Read the model definition and answer for the solid it produces. Units are mm, in the model's axes. Face numbers are marked on the shaded views. A direction names the side the tool comes from. Coordinates: 2 decimals unless noted, no trailing zeros. Loops run counter-clockwise (first coordinate to the right, second up) from the corner with the lowest first, then second, coordinate; pieces in that order, holes last.
Autodesk Inventor part; units mm, degrees
ref_plane "YZ Plane" through (0, 0, 0) normal (1, 0, 0) x (0, 1, 0)
ref_plane "XZ Plane" through (0, 0, 0) normal (0, 1, 0) x (-1, 0, 0)
ref_plane "XY Plane" through (0, 0, 0) normal (0, 0, 1) x (1, 0, 0)
sketch "Sketch1" plane through (0, 0, 0) normal (0, 0, 1) x (1, 0, 0)
  line L0 (20.1195, -38.0715) -> (-17.9805, -38.0715)
  line L1 (-17.9805, -38.0715) -> (-17.9805, -114.2715)
  line L2 (-17.9805, -114.2715) -> (20.1195, -114.2715)
  line L3 (20.1195, -114.2715) -> (20.1195, -38.0715)
  line L4 (16.9445, -111.0965) -> (-14.8055, -111.0965)
  line L5 (-14.8055, -111.0965) -> (-14.8055, -41.2465)
  line L6 (-14.8055, -41.2465) -> (16.9445, -41.2465)
  line L7 (16.9445, -41.2465) -> (16.9445, -111.0965)
  point P0 (0, 0)
  dimension "d0" = 76.2
  dimension "d1" = 38.1
  dimension "d2" = 3.175
extrude "Extrusion1" add sketch "Sketch1" along normal blind 130.175
sketch "Sketch2" plane through (-17.9805, -114.2715, 0) normal (-1, 0, 0) x (0, 0, 1)
  line L0 (0, 76.2) -> (130.175, 76.2)
  line L1 (0, 76.2) -> (0, 0)
  line L2 (0, 0) -> (130.175, 0)
  line L3 (130.175, 76.2) -> (130.175, 0)
  line L4 (130.175, 76.2) -> (38.1, 76.2)
  line L5 (38.1, 76.2) -> (38.1, 38.1)
  line L6 (38.1, 38.1) -> (130.175, 38.1)
  line L7 (130.175, 38.1) -> (130.175, 76.2)
  point P0 (0, 114.2715)
  dimension "d25" = 38.1
  dimension "d26" = 38.1
extrude "Extrusion2" cut sketch "Sketch2" against normal blind 19.05 contours L0 L3 L6 L5
sketch "Sketch3" plane through (-17.9805, -114.2715, 0) normal (0, -1, 0) x (1, 0, 0)
  line L0 (38.1, 0) -> (38.1, 130.175)
  line L1 (0, 130.175) -> (38.1, 130.175)
  point P0 (17.9805, 0)
  point P1 (25.4, 121.285)
  point P2 (25.4, 108.585)
  point P3 (25.4, 95.885)
  point P4 (25.4, 83.185)
  point P5 (25.4, 70.485)
  point P6 (25.4, 57.785)
  point P7 (25.4, 45.085)
  point P8 (25.4, 32.385)
  point P9 (25.4, 19.685)
  point P10 (25.4, 6.985)
  dimension "d9" = 12.7
  dimension "d10" = 8.89
  dimension "d13" = 12.7
hole "Hole1" at (7.4195, -114.2715, 121.285) at (7.4195, -114.2715, 108.585) at (7.4195, -114.2715, 95.885) at (7.4195, -114.2715, 83.185) at (7.4195, -114.2715, 70.485) at (7.4195, -114.2715, 57.785) at (7.4195, -114.2715, 45.085) at (7.4195, -114.2715, 32.385) at (7.4195, -114.2715, 19.685) at (7.4195, -114.2715, 6.985) direction (0, 1, 0) diameter 6.35 end through all
properties part number "2018 Scissor Stand Off Outside A"
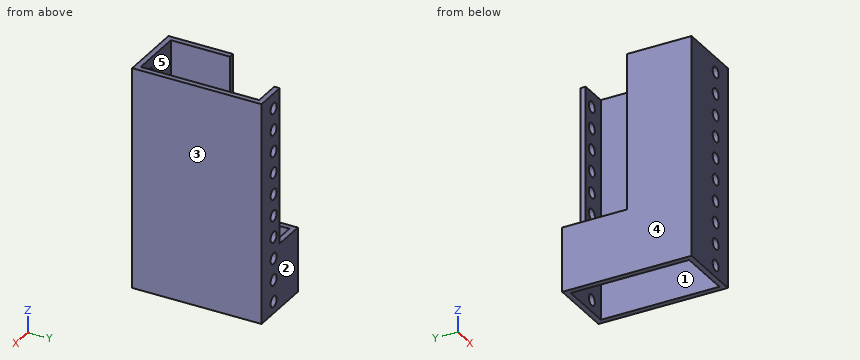
Item 1: A cutting plane is placed at A-A on y = -101. Determine the outline of the cut face in (x, z) (1 decimal).
Numbers:
outline: (-18, 0) - (-14.8, 0) - (-14.8, 130.2) - (-18, 130.2) - close; (16.9, 0) - (20.1, 0) - (20.1, 130.2) - (16.9, 130.2) - close
Item 2: A cutting plane is placed at B-B on x = -7.5. Determine the outline of the cut face in (y, z) (1 decimal).
Numbers:
outline: (-114.3, 0) - (-111.1, 0) - (-111.1, 130.2) - (-114.3, 130.2) - close; (-41.2, 0) - (-38.1, 0) - (-38.1, 38.1) - (-41.2, 38.1) - close
Item 3: Which of the six approach directions +Z, -Z, +X, -X, +Y, -Y give full straight-line access (tool end or side, diameter ignored) to the marked faces 4 and 5?
Numbers:
face 4: +Z, -Z, -X, +Y, -Y
face 5: +Z, -Z
Item 4: A cutting plane is placed at C-C on z = 47. Determine the outline of the cut face in (x, y), then the cut area to 3 significant figures.
Numbers:
outline: (-17.98, -114.27) - (4.89, -114.27) - (4.89, -111.1) - (-14.81, -111.1) - (-14.81, -76.17) - (-17.98, -76.17) - close; (1.07, -41.25) - (4.89, -41.25) - (4.89, -38.07) - (1.07, -38.07) - close; (9.95, -114.27) - (20.12, -114.27) - (20.12, -38.07) - (9.95, -38.07) - (9.95, -41.25) - (16.94, -41.25) - (16.94, -111.1) - (9.95, -111.1) - close
area: 482 mm2
Item 5: A cutting plane is placed at D-D on z = 96. Determine the outline of the cut face in (x, y).
Numbers:
outline: (-17.98, -114.27) - (4.25, -114.27) - (4.25, -111.1) - (-14.81, -111.1) - (-14.81, -76.17) - (-17.98, -76.17) - close; (1.07, -41.25) - (4.25, -41.25) - (4.25, -38.07) - (1.07, -38.07) - close; (10.59, -114.27) - (20.12, -114.27) - (20.12, -38.07) - (10.59, -38.07) - (10.59, -41.25) - (16.94, -41.25) - (16.94, -111.1) - (10.59, -111.1) - close
Item 6: Determine the mould class of the marked faces 1, 2 and 3 for opening direction X: released by +X, released by -X, zero draft, split by the parting line, or undercut.
Numbers:
face 1: undercut
face 2: zero draft
face 3: released by +X
Item 7: Given pin 1 (5.5 mm diameter, centred on x = 7.42, z = 6.98, fed in from -Y), flat-ended and moving along its own axis, determine where the tip first touches the part or whether it passes through.
Numbers:
pin 1: passes through
Item 8: Find the intervals of material crossed by line 1 along Y through (x, z) = (14, 82); line 2 along X through (y, z) = (-42.5, 30.5); line 3 along Y through (x, z) = (-11.5, 74), in increasing order.
Numbers:
line 1: y = -114.27 to -111.1, -41.25 to -38.07
line 2: x = -17.98 to -14.81, 16.94 to 20.12
line 3: y = -114.27 to -111.1
